from build123d import *

# Parameters (mm, degrees)
SKETCH1_W           = 50
SKETCH1_H           = 60
BOSS_EXTRUDE1_DEPTH = 2
SKETCH2_W           = 15
SKETCH2_H           = 20
SKETCH2_H_2         = 14
BOSS_EXTRUDE2_DEPTH = 5
SKETCH3_R           = 2.5
CUT_EXTRUDE1_DEPTH  = 7
SKETCH4_W           = 10
SKETCH4_H           = 16.5
SKETCH4_R           = 2.5
BOSS_EXTRUDE3_DEPTH = 2
SKETCH5_W           = 10
SKETCH5_H           = 16.5
SKETCH5_R           = 2.5
BOSS_EXTRUDE5_DEPTH = 3.8


with BuildPart() as part:
    # Sketch1 → Boss-Extrude1 (new body)
    with BuildSketch(Plane(origin=(0, 0, 0), x_dir=(1, 0, 0), z_dir=(0, 1, 0))):
        with Locations((25, 30)):
            Rectangle(SKETCH1_W, SKETCH1_H)
    extrude(amount=BOSS_EXTRUDE1_DEPTH)

    # Sketch2 → Boss-Extrude2 (add)
    with BuildSketch(Plane.XZ):
        with Locations((42.5, -10)):
            Rectangle(SKETCH2_W, SKETCH2_H)
        with Locations((7.5, -53)):
            Rectangle(SKETCH2_W, SKETCH2_H_2)
    extrude(amount=BOSS_EXTRUDE2_DEPTH)

    # Sketch3 → Cut-Extrude1 (cut)
    with BuildSketch(Plane(origin=(0, 2, 0), x_dir=(1, 0, 0), z_dir=(0, 1, 0))):
        with Locations(Location((45, 5, 0), (0, 0, 270))):
            Circle(SKETCH3_R)
        with Locations(Location((5, 55, 0), (0, 0, 270))):
            Circle(SKETCH3_R)
    extrude(amount=-CUT_EXTRUDE1_DEPTH, mode=Mode.SUBTRACT)

    # Sketch4 → Boss-Extrude3 (add)
    # profile 1 of 2: a face of its own
    with BuildSketch(Plane(origin=(0, 2, 0), x_dir=(1, 0, 0), z_dir=(0, 1, 0))):
        with Locations((9, 68.25)):
            Rectangle(SKETCH4_W, SKETCH4_H)
        with Locations(Location((9, 71.5, 0), (0, 0, 270))):
            Circle(SKETCH4_R, mode=Mode.SUBTRACT)
    # profile 2 of 2: a face of its own
    with BuildSketch(Plane(origin=(0, 2, 0), x_dir=(1, 0, 0), z_dir=(0, 1, 0))):
        with Locations((9, -8.25)):
            Rectangle(SKETCH4_W, SKETCH4_H)
        with Locations(Location((9, -11.5, 0), (0, 0, 270))):
            Circle(SKETCH4_R, mode=Mode.SUBTRACT)
    extrude(amount=-BOSS_EXTRUDE3_DEPTH)

    # Sketch5 → Boss-Extrude5 (add)
    # profile 1 of 2: a face of its own
    with BuildSketch(Plane(origin=(0, 2, 0), x_dir=(1, 0, 0), z_dir=(0, 1, 0))):
        with Locations((31, 68.25)):
            Rectangle(SKETCH5_W, SKETCH5_H)
        with Locations(Location((31, 71.5, 0), (0, 0, 270))):
            Circle(SKETCH5_R, mode=Mode.SUBTRACT)
    # profile 2 of 2: a face of its own
    with BuildSketch(Plane(origin=(0, 2, 0), x_dir=(1, 0, 0), z_dir=(0, 1, 0))):
        with Locations((31, -8.25)):
            Rectangle(SKETCH5_W, SKETCH5_H)
        with Locations(Location((31, -11.5, 0), (0, 0, 270))):
            Circle(SKETCH5_R, mode=Mode.SUBTRACT)
    extrude(amount=-BOSS_EXTRUDE5_DEPTH)


solid = part.part
Could you check a few things on this model? Use its own coordinates, in mm. A direction names the side the tool comes from. Coordinates: 2 decimals unless noted, no trailing zeros. Write each loop counter-clockwise with the first axis right and the second up, starting at its lowest first coordinate (ties: lowest second). Pieces come first, ordered by that corner, then holes. Notation, with made-up numbers: (-40, -34) - (1, -34) arc R5 cw to (1, -29) - close; hole circle Ø4 at (44.5, -25). An arc over 180 degrees is marked (long way). Write item = value, one per line.
1) Suppose I cut it at C-C on z = -53.5. Please give me the cut outline in (x, y), plus the area to 3 significant figures.
Result set:
outline = (0, -5) - (3, -5) - (3, 2) - (0, 2) - close; (7, -5) - (15, -5) - (15, 0) - (50, 0) - (50, 2) - (7, 2) - close
area = 147 mm2
2) Suppose I cut it at D-D on z = 11.5. Please give me the cut outline in (x, y), plus the area to 3 significant figures.
Result set:
outline = (4, 0) - (6.5, 0) - (6.5, 2) - (4, 2) - close; (11.5, 0) - (14, 0) - (14, 2) - (11.5, 2) - close; (26, -1.8) - (28.5, -1.8) - (28.5, 2) - (26, 2) - close; (33.5, -1.8) - (36, -1.8) - (36, 2) - (33.5, 2) - close
area = 29.0 mm2
3) We'd pull the mould along Z, two halves only. Please class faces 6 (the flat face through (35, -2, -10)), 7 (the flat face through (42, -5, -10)), 8 (the flat face through (9, 1, -76.5)): +Z half, -Z half, draft (parallel to the pull), parting line (faces both ways), or undercut.
Result set:
face_6 = undercut
face_7 = draft
face_8 = -Z half
4) For faces 1 (the flat face through (31, -1.8, 8)), 2 (the flat face through (0, 1, -36)), 3 (the flat face through (20, 1, 0)), 4 (the flat face through (2, 1, 0)), 5 (the flat face through (14, 1, -68)), which set-ups out of +Z, -Z, +X, -X, +Y, -Y let a thin tool reach every point of the face, with its end or its side?
Result set:
face_1 = +Z, +X, -X, -Y
face_2 = +Z, -Z, -X, +Y, -Y
face_3 = +Z, +Y, -Y
face_4 = +Z, -X, +Y, -Y
face_5 = -Z, +Y, -Y
5) Will these pins go through, and if not, where does the flat tip stop? pin 1 Ø1.1 at (y, z) = (1, 6.5) entering from -X; pin 2 Ø4.5 at (x, z) = (5, -55) entering from +Y; pin 3 Ø2.5 at (y, z) = (-2, -6) entering from -X; pin 4 Ø1.5 at (x, z) = (18, -36) entering from -Y.
Result set:
pin_1 = 4
pin_2 = through
pin_3 = 35
pin_4 = 0
6) Suppose I cut it at A-A on y = -3. Please give me the cut outline in (x, z).
Result set:
outline = (0, -60) - (15, -60) - (15, -46) - (0, -46) - close; (35, -20) - (50, -20) - (50, 0) - (35, 0) - close; hole circle Ø5 at (5, -55); hole circle Ø5 at (45, -5)
7) Please list where these lines run through material, in increasing order: line 1 (X direction, y = 0.85, z = -71.5); line 2 (X direction, y = -1.75, z = -55); line 3 (X direction, y = -0.5, z = -5). Write a range as [from, to].
Result set:
line_1 = [4, 6.5], [11.5, 14], [26, 28.5], [33.5, 36]
line_2 = [0, 2.5], [7.5, 15]
line_3 = [35, 42.5], [47.5, 50]
8) Suppose I cut it at B-B on x = 9. Please give me the cut outline in (y, z), plus the area to 3 significant figures.
Result set:
outline = (-5, -60) - (0, -60) - (0, -69) - (2, -69) - (2, 9) - (0, 9) - (0, -46) - (-5, -46) - close; (0, -76.5) - (2, -76.5) - (2, -74) - (0, -74) - close; (0, 14) - (2, 14) - (2, 16.5) - (0, 16.5) - close
area = 236 mm2
